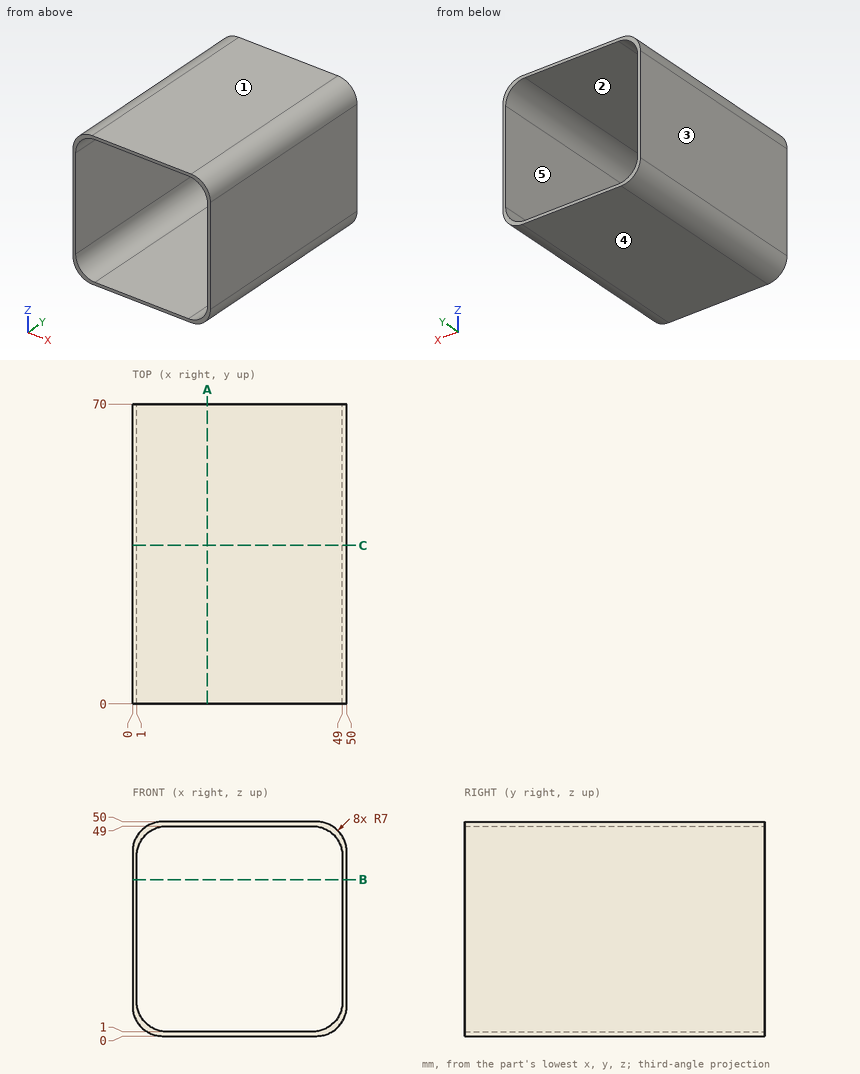
Study the drawing (mm; zero at the part's minimum x, y, z) and answer. A direction names the side the tool comes from. Give positions to 0.01 mm unless a question says otherwise; leave off trailing zeros. Loops run counter-clockwise (first coordinate to the right, second up) from the corner with the lowest first, then second, coordinate; pieces in that order, holes last. Notation, with made-up numbers: M -1.75,-25.5 L 20.25,-25.5 A24 cw 20.25,-5.5 Z; hole C 54,31 d10. An arc over 180 degrees is marked long. Answer as CSV lines item,"result".
Item 1: The part is cut by section C-C (y = 37). Give the vertices of the cut face in (x, z), and give its area (3 significant figures).
Values follow:
outline,"M 0,7 A7 ccw 7,0 L 43,0 A7 ccw 50,7 L 50,43 A7 ccw 43,50 L 7,50 A7 ccw 0,43 Z; hole M 1,8 A7 ccw 8,1 L 42,1 A7 ccw 49,8 L 49,42 A7 ccw 42,49 L 8,49 A7 ccw 1,42 Z"
area,"196 mm^2"
Item 2: Straight lines are drawn through the part: line 1 along X through (y, z) = (33.5, 12.5); line 2 along Z through (x, y) = (47.5, 12). For each, find the intervals that lie inside material, in ascending order. Write a range as [from, to].
Values follow:
line 1,"x = [0, 1], [49, 50]"
line 2,"z = [1.64, 3.67], [46.33, 48.36]"
Item 3: The part is cut by section A-A (x = 17.5). Give the vertices of the cut face in (y, z), and give its area (3 significant figures).
Values follow:
outline,"M 0,0 L 70,0 L 70,1 L 0,1 Z; M 0,49 L 70,49 L 70,50 L 0,50 Z"
area,"140 mm^2"
Item 4: Which of the six approach directions +Z, -Z, +X, -X, +Y, -Y give full straight-line access (tool end or side, diameter ignored) to the marked faces 1 and 2?
Values follow:
face 1,"+Z, +X, -X, +Y, -Y"
face 2,"+Y, -Y"
Item 5: The part is cut by section B-B (z = 36.5). Give the vertices of the cut face in (x, y), and give its area (3 significant figures).
Values follow:
outline,"M 0,0 L 1,0 L 1,70 L 0,70 Z; M 49,0 L 50,0 L 50,70 L 49,70 Z"
area,"140 mm^2"
Item 6: The mould has two halves that part along X. Classify the marked faces 3, 4 and 5: released by +X, released by -X, zero draft, split by the parting line, or undercut.
Values follow:
face 3,"released by -X"
face 4,"zero draft"
face 5,"undercut"
